Input: part model. Units: mm. Frame: model coordinates. A direction names the side the tool comes from. Coordinates: 2 decimals unless noted, no trailing zeros. Loops run counter-clockwise (first coordinate to the right, second up) from the corner with the lowest first, then second, coordinate; pieces in that order, holes last.
(1) Line query: L1, parallel to Y at x = 14.5, z = 10; L2, parallel to Y at x = 16.75, z = 10; L3, parallel to X at y = 29, z = 2. Output: solid intervals per line, ascending.
(2) Section B-B, the plane y = -8. Return loops of the section in (x, z), then the cut area to 3 significant figures.
(3) Contact query for flat-ended pins moving along their axis: P1, Ø4, axis at y = -23, z = 10, coming from the +X side; P2, Ø1.5, axis at y = -13.5, z = 13.5, coming from the -X side; P3, Ø2, axis at x = 14.5, z = 11.5, coming from the +Y side; P4, Ø11, axis at x = 3.5, z = 5, coming from the -Y side. Output: stop coordinate, or through.
(4) Section C-C, the plane z = 15.5. Return loops of the section in (x, y), then the cut area to 3 significant figures.
(5) Section A-A, the plane z = 10. Return loops of the section in (x, y), then the cut area to 3 significant figures.
(6) Section D-D, the plane x = 17.5. Return loops of the section in (y, z), then the cut area to 3 significant figures.
(7) Set-up query: faces 1 (the face through (5, 0, 10)), 2 (the face through (10, 57, 10)), 3 (the face through (20, -12, 10)). Return all of +Z, -Z, +X, -X, +Y, -Y with unobstructed straight access to the full face (end or side cutting, diameter ignored); none if empty.
```python
from build123d import *

# Parameters (mm, degrees)
BOSS_EXTRUDE1_DEPTH = 20
SKETCH2_R           = 2.5
CUT_EXTRUDE1_DEPTH  = 21
FILLET1_R           = 3


with BuildPart() as part:
    # Sketch1 → Boss-Extrude1 (new body)
    with BuildSketch(Plane.XY):
        with BuildLine():
            Line((0, 0), (10, 0))
            Line((10, 0), (10, -29))
            Line((10, -29), (20, -29))
            Line((20, -29), (20, 6))
            ThreePointArc((20, 6), (18.828427125, 8.828427125), (16, 10))
            Line((16, 10), (14, 10))
            ThreePointArc((14, 10), (11.171572875, 11.171572875), (10, 14))
            Line((10, 14), (10, 100.857864376))
            ThreePointArc((10, 100.857864376), (8.15587029, 108.063631297), (3.076923077, 113.497615703))
            ThreePointArc((3.076923077, 113.497615703), (1.039231077, 113.566431565), (0, 111.812315526))
            Line((0, 111.812315526), (0, 0))
        make_face()
    extrude(amount=BOSS_EXTRUDE1_DEPTH)

    # Sketch2 → Cut-Extrude1 (cut, through all)
    with BuildSketch(Plane(origin=(20, 0, 0), x_dir=(0, 0, -1), z_dir=(1, 0, 0))):
        with Locations((-10, -8)):
            Circle(SKETCH2_R)
        with Locations((-10, -23)):
            Circle(SKETCH2_R)
    extrude(amount=-CUT_EXTRUDE1_DEPTH, mode=Mode.SUBTRACT)

    # Fillet1
    fillet1_edges = [part.edges().sort_by_distance(p)[0] for p in [
        (10, -29, 10),
    ]]
    fillet(fillet1_edges, radius=FILLET1_R)


solid = part.part
```
Report:
1. L1: y = -29 to -25.5, -20.5 to -10.5, -5.5 to 10
1. L2: y = -29 to -25.5, -20.5 to -10.5, -5.5 to 9.93
1. L3: x = 0 to 10
2. outline: (10, 0) - (20, 0) - (20, 7.5) - (10, 7.5) - close; (10, 12.5) - (20, 12.5) - (20, 20) - (10, 20) - close
2. area: 150 mm2
3. P1: passes through
3. P2: stops at x = 10
3. P3: stops at y = 10.03
3. P4: stops at y = 0
4. outline: (0, 0) - (10, 0) - (10, -26) arc R3 ccw to (13, -29) - (20, -29) - (20, 6) arc R4 ccw to (16, 10) - (14, 10) arc R4 cw to (10, 14) - (10, 100.86) arc R15 ccw to (3.08, 113.5) arc R2 ccw to (0, 111.81) - close
4. area: 1,500 mm2
5. outline: (0, 0) - (10, 0) - (10, -5.5) - (20, -5.5) - (20, 6) arc R4 ccw to (16, 10) - (14, 10) arc R4 cw to (10, 14) - (10, 100.86) arc R15 ccw to (3.08, 113.5) arc R2 ccw to (0, 111.81) - close; (10, -26) arc R3 ccw to (13, -29) - (20, -29) - (20, -25.5) - (10, -25.5) - close; (10, -20.5) - (20, -20.5) - (20, -10.5) - (10, -10.5) - close
5. area: 1,400 mm2
6. outline: (-29, 0) - (9.71, 0) - (9.71, 20) - (-29, 20) - close; hole circle Ø5 at (-23, 10); hole circle Ø5 at (-8, 10)
6. area: 735 mm2
7. face 1: +Z, -Z, -X, -Y
7. face 2: +Z, -Z, +X, +Y
7. face 3: +Z, -Z, +X, +Y, -Y
